Source: CAD feature listing. Evaluate the final solid. Frame: model axes, mm. Face numbers are marked on the shaded views. A direction names the side the tool comes from. Give positions to 0.01 mm unless a question says otherwise; leave off trailing zeros. Write each loop counter-clockwise with the first axis right and the second up, starting at its lowest first coordinate (ties: lowest second). Pieces come first, ordered by that corner, then holes.
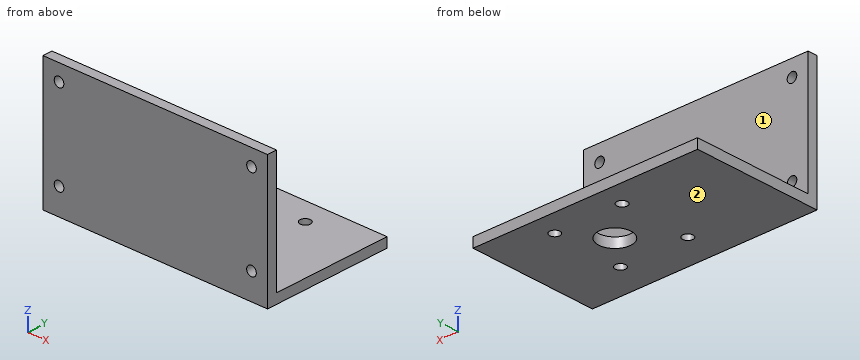
```python
from build123d import *

# Parameters (mm, degrees)
EXTRUDE_1_DEPTH     = 70
SKETCH_2_R          = 5
SKETCH_2_R_2        = 1.6
CUT_EXTRUDE_1_DEPTH = 3
SKETCH_3_R          = 1.5
CUT_EXTRUDE_2_DEPTH = 3


with BuildPart() as part:
    # Эскиз1 → Бобышка-Вытянуть1 (new body)
    with BuildSketch(Plane(origin=(0, 0, 0), x_dir=(0, 0, -1), z_dir=(1, 0, 0))):
        Polygon((17, -17), (-20, -17), (-20, -20), (20, -20), (20, 20), (17, 20), align=None)
    extrude(amount=EXTRUDE_1_DEPTH)

    # Эскиз2 → Вырез-Вытянуть1 (cut)
    with BuildSketch(Plane.XY.offset(-17)):
        with Locations((43, 1.5)):
            Circle(SKETCH_2_R)
        with Locations((51.5, 12.5)):
            Circle(SKETCH_2_R_2)
        with Locations((30.5, 12.5)):
            Circle(SKETCH_2_R_2)
        with Locations((30.5, -9.5)):
            Circle(SKETCH_2_R_2)
        with Locations((51.5, -9.5)):
            Circle(SKETCH_2_R_2)
    extrude(amount=-CUT_EXTRUDE_1_DEPTH, mode=Mode.SUBTRACT)

    # Эскиз3 → Вырез-Вытянуть2 (cut)
    with BuildSketch(Plane(origin=(0, -17, 0), x_dir=(1, 0, 0), z_dir=(0, 1, 0))):
        with Locations(Location((65, -15, 0), (0, 0, 270))):
            Circle(SKETCH_3_R)
        with Locations(Location((65, 12, 0), (0, 0, 270))):
            Circle(SKETCH_3_R)
        with Locations(Location((5, -15, 0), (0, 0, 270))):
            Circle(SKETCH_3_R)
        with Locations(Location((5, 12, 0), (0, 0, 270))):
            Circle(SKETCH_3_R)
    extrude(amount=-CUT_EXTRUDE_2_DEPTH, mode=Mode.SUBTRACT)


solid = part.part
```
1. Line query: L1, parallel to X at y = -18, z = 15; L2, parallel to X at y = 12, z = -18; L3, parallel to Y at x = 54.5, z = 6. Output: solid intervals per line, ascending.
2. Cut plane C-C, the plane y = -9.5. Return the cut outline in (x, z), then the cut area to 3 significant figures.
3. Access query for the marked faces 1 and 2. Directions: +Z, -Z, +X, -X, +Y, -Y. A direction counts if a zero-diameter tool reaches every point of the face in a straight line with its end or side. Return the directions, or none.
4. Cut plane B-B, the plane x = 51.5. Return the cut outline in (y, z), then the cut area to 3 significant figures.
5. Contact query for flat-ended pins moving along their axis: P1, Ø5, axis at x = 51.5, y = 12.5, coming from the +Z side; P2, Ø5, axis at x = 5, z = 15, coming from the +Y side. Output: stop coordinate, or through.
6. Cut plane A-A, the plane y = 1.5. Return the cut outline in (x, z).
7. Cut plane D-D, the plane z = -12. Return the cut outline in (x, y).
Response values:
1. L1: x = 0 to 3.5, 6.5 to 63.5, 66.5 to 70
1. L2: x = 0 to 28.98, 32.02 to 49.98, 53.02 to 70
1. L3: y = -20 to -17
2. outline: (0, -20) - (28.9, -20) - (28.9, -17) - (0, -17) - close; (32.1, -20) - (49.9, -20) - (49.9, -17) - (32.1, -17) - close; (53.1, -20) - (70, -20) - (70, -17) - (53.1, -17) - close
2. area: 191 mm2
3. face 1: +Z, +X, -X, +Y
3. face 2: -Z, +X, -X, +Y, -Y
4. outline: (-20, -20) - (-11.1, -20) - (-11.1, -17) - (-17, -17) - (-17, 20) - (-20, 20) - close; (-7.9, -20) - (10.9, -20) - (10.9, -17) - (-7.9, -17) - close; (14.1, -20) - (20, -20) - (20, -17) - (14.1, -17) - close
4. area: 212 mm2
5. P1: stops at z = -17
5. P2: stops at y = -17
6. outline: (0, -20) - (38, -20) - (38, -17) - (0, -17) - close; (48, -20) - (70, -20) - (70, -17) - (48, -17) - close
7. outline: (0, -20) - (3.5, -20) - (3.5, -17) - (0, -17) - close; (6.5, -20) - (63.5, -20) - (63.5, -17) - (6.5, -17) - close; (66.5, -20) - (70, -20) - (70, -17) - (66.5, -17) - close
